from build123d import *

# Parameters (mm, degrees)
SKETCH1_W           = 25.4
SKETCH1_H           = 7.62
SKETCH1_R           = 0.5
BOSS_EXTRUDE1_DEPTH = 1.6
SKETCH2_R           = 0.9
SKETCH2_R_2         = 0.49
BOSS_EXTRUDE2_DEPTH = 1.62
SKETCH3_W           = 4.3
SKETCH3_H           = 6.04
BOSS_EXTRUDE3_DEPTH = 3.16
CUT_EXTRUDE1_DEPTH  = 3.5


with BuildPart() as part:
    # Sketch1 → Boss-Extrude1 (new body)
    with BuildSketch(Plane(origin=(0, 0, 0), x_dir=(1, 0, 0), z_dir=(0, 1, 0))):
        Rectangle(SKETCH1_W, SKETCH1_H)
        with Locations(Location((-3.81, 1.27, 0), (0, 0, 270))):
            Circle(SKETCH1_R, mode=Mode.SUBTRACT)
        with Locations(Location((-1.27, 1.27, 0), (0, 0, 270))):
            Circle(SKETCH1_R, mode=Mode.SUBTRACT)
        with Locations(Location((1.27, 1.27, 0), (0, 0, 270))):
            Circle(SKETCH1_R, mode=Mode.SUBTRACT)
        with Locations(Location((3.81, 1.27, 0), (0, 0, 270))):
            Circle(SKETCH1_R, mode=Mode.SUBTRACT)
    extrude(amount=BOSS_EXTRUDE1_DEPTH)

    # Sketch2 → Boss-Extrude2 (add)
    # profile 1 of 4: a face of its own
    with BuildSketch(Plane(origin=(0, 1.61, 0), x_dir=(1, 0, 0), z_dir=(0, 1, 0))):
        with Locations(Location((-3.81, 1.27, 0), (0, 0, 270))):
            Circle(SKETCH2_R)
        with Locations(Location((-3.81, 1.27, 0), (0, 0, 270))):
            Circle(SKETCH2_R_2, mode=Mode.SUBTRACT)
    # profile 2 of 4: a face of its own
    with BuildSketch(Plane(origin=(0, 1.61, 0), x_dir=(1, 0, 0), z_dir=(0, 1, 0))):
        with Locations(Location((1.27, 1.27, 0), (0, 0, 270))):
            Circle(SKETCH2_R)
        with Locations(Location((1.27, 1.27, 0), (0, 0, 270))):
            Circle(SKETCH2_R_2, mode=Mode.SUBTRACT)
    # profile 3 of 4: a face of its own
    with BuildSketch(Plane(origin=(0, 1.61, 0), x_dir=(1, 0, 0), z_dir=(0, 1, 0))):
        with Locations(Location((-1.27, 1.27, 0), (0, 0, 270))):
            Circle(SKETCH2_R)
        with Locations(Location((-1.27, 1.27, 0), (0, 0, 270))):
            Circle(SKETCH2_R_2, mode=Mode.SUBTRACT)
    # profile 4 of 4: a face of its own
    with BuildSketch(Plane(origin=(0, 1.61, 0), x_dir=(1, 0, 0), z_dir=(0, 1, 0))):
        with Locations(Location((3.81, 1.27, 0), (0, 0, 270))):
            Circle(SKETCH2_R)
        with Locations(Location((3.81, 1.27, 0), (0, 0, 270))):
            Circle(SKETCH2_R_2, mode=Mode.SUBTRACT)
    extrude(amount=-BOSS_EXTRUDE2_DEPTH)

    # Sketch3 → Boss-Extrude3 (add)
    with BuildSketch(Plane(origin=(0, 1.6, 0), x_dir=(1, 0, 0), z_dir=(0, 1, 0))):
        with Locations((-10.54, 0)):
            Rectangle(SKETCH3_W, SKETCH3_H)
        with Locations((10.54, 0)):
            Rectangle(SKETCH3_W, SKETCH3_H)
    extrude(amount=BOSS_EXTRUDE3_DEPTH)

    # Sketch4 → Cut-Extrude1 (cut)
    with BuildSketch(Plane.ZY.offset(12.69)):
        Polygon((2.27, 4.46), (-2.27, 4.46), (-2.27, 3.56), (-2.72, 3.56), (-2.72, 2.81), (-2.27, 2.81), (-2.27, 1.91), (2.27, 1.91), (2.27, 2.81), (2.72, 2.81), (2.72, 3.56), (2.27, 3.56), align=None)
    cut_extrude1 = extrude(amount=-CUT_EXTRUDE1_DEPTH, mode=Mode.SUBTRACT)

    # Mirror1: Cut-Extrude1 across plane
    add(cut_extrude1.mirror(Plane(origin=(0, 0, 0), x_dir=(0, 0, 1), z_dir=(1, 0, 0))), mode=Mode.SUBTRACT)


solid = part.part
Geometry: final body of the model. Coordinates: model frame, mm. A direction names the side the tool comes from. Round coordinates to 2 decimals unless told otherwise and drop trailing zeros. Write item = value, one per line.
Item 1: Access query for faces 1 (the face through (11, 3, 3.02)), 2 (the face through (-11, 4, 2.27)), 3 (the face through (11, 2.4, -2.27)). Directions: +Z, -Z, +X, -X, +Y, -Y. A direction counts if a zero-diameter tool reaches every point of the face in a straight line with its end or side. Return the directions, or none.
Findings:
face_1 = +Z, +X, -X, +Y
face_2 = -X
face_3 = +X
Item 2: Pin query (flat end, axial travel): P1, Ø1.5, axis at y = 3, z = 0.5, coming from the -X side; P2, Ø1.6, axis at x = -10.5, y = 3.5, coming from the -Z side; P3, Ø2.5, axis at x = -11, y = 3, coming from the +Z side. Return the tip coordinate at first contact, or that it passes through.
Findings:
P1 = -9.19
P2 = -3.02
P3 = 3.02
Item 3: Section query B-B on z = -1.27. State how many separate pieces and enclosed holes the cut face has, then the cut area to 3 significant figures.
Findings:
separate_pieces = 5
enclosed_holes = 0
area = 43.8 mm^2
Item 4: Material intervals for line 1 along X through (y, z) = (1, -1.27); line 2 along X through (y, z) = (4.25, 1.25); line 3 along Y through (x, z) = (-9.75, 0), sorted ascending. Write a range as [from, to].
Findings:
line_1 = [-12.7, -4.3], [-3.32, -1.76], [-0.78, 0.78], [1.76, 3.32], [4.3, 12.7]
line_2 = [-9.19, -8.39], [8.39, 9.19]
line_3 = [0, 1.91], [4.46, 4.76]
Item 5: Pull-direction query (X, two-part tool) for faces 4 (the face through (-1.568, 0.811, -1.659)), 5 (the face through (11, 4.76, 0)); classes: pulls with the +X half, pulls with the -X half, needs draft (parallel to the pull), parting line crosses it, or undercut.
Findings:
face_4 = undercut
face_5 = needs draft
